Geometry: final body of the model. Coordinates: model frame, mm. Round coordinates to 2 decimals unless told otherwise and drop trailing zeros. Loops run counter-clockwise (first coordinate to the right, second up) from the corner with the lowest first, then second, coordinate; pieces in that order, holes last. Notation, with made-up numbers: (41.5, 43) - (89.5, 43) arc R25 ccw to (89.5, 61) - close; hole circle Ø9 at (36, 44.25). An arc over 180 degrees is marked (long way). Answer as a JSON object with one key per item and string values. Group by question number.
Item 1: Line query: line 1 (X direction, y = 5, z = 1310); line 2 (Y direction, x = 20, z = 30). Output: solid intervals per line, ascending.
Item 2: Section C-C (x = 21). Return the cut outline in (y, z).
Item 3: First-contact query: pin 1 (22 mm diameter, centred on x = 21, z = 489, fed in from -Y). Flat tip, straight axial feed; report the tip coordinate or a pass-through.
Item 4: Section B-B (z = 446). Return the cut outline in (x, y), plus the area to 3 significant figures.
Item 5: Section A-A (y = 7.5). Return the cut outline in (x, z), plus the area to 3 significant figures.
```python
from build123d import *

# Parameters (mm, degrees)
BOSS_EXTRUDE1_DEPTH = 1785
EXTRUDE_R_DEPTH     = 60
EXTRUDE_L_DEPTH     = 60


with BuildPart() as part:
    # Sketch1 → Boss-Extrude1 (new body)
    with BuildSketch(Plane.XY):
        Polygon((0, 0), (0, 20), (50, 20), (50, 0), (47, 0), (47, 17), (3, 17), (3, 0), align=None)
    extrude(amount=BOSS_EXTRUDE1_DEPTH)

    # Sketch2 → Extrude R (add)
    with BuildSketch(Plane.XY.offset(1785)):
        Polygon((0, 0), (0, 20), (50, 20), (50, 0), (47, 0), (47, 17), (3, 17), (3, 0), align=None)
    extrude(amount=EXTRUDE_R_DEPTH)

    # Sketch3 → Extrude L (add)
    with BuildSketch(Plane(origin=(0, 0, 0), x_dir=(-1, 0, 0), z_dir=(0, 0, -1))):
        Polygon((-50, 0), (-50, 20), (0, 20), (0, 0), (-3, 0), (-3, 17), (-47, 17), (-47, 0), align=None)
    extrude(amount=EXTRUDE_L_DEPTH)


solid = part.part
```
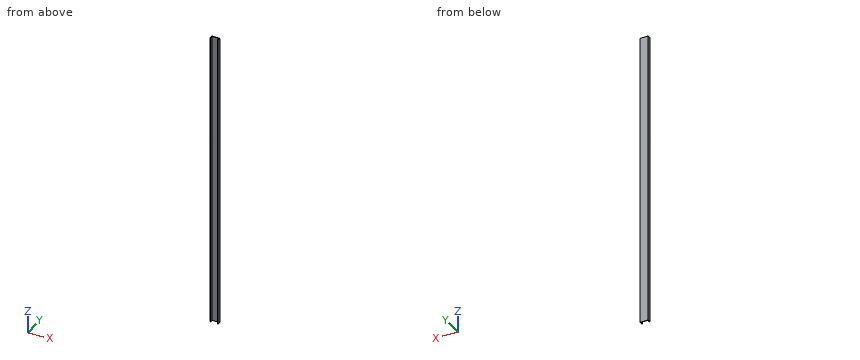
Values:
{
 "1": {"line 1": "x = 0 to 3, 47 to 50", "line 2": "y = 17 to 20"},
 "2": {"outline": "(17, -60) - (20, -60) - (20, 1845) - (17, 1845) - close"},
 "3": {"pin 1": "stops at y = 17"},
 "4": {"outline": "(0, 0) - (3, 0) - (3, 17) - (47, 17) - (47, 0) - (50, 0) - (50, 20) - (0, 20) - close", "area": "252 mm^2"},
 "5": {"outline": "(0, -60) - (3, -60) - (3, 1845) - (0, 1845) - close; (47, -60) - (50, -60) - (50, 1845) - (47, 1845) - close", "area": "11,400 mm^2"}
}
